Could you check a few things on this model? Use its own coordinates, in mm. Face numbers are marked on the shaded views. Round coordinates to 2 decimals unless told otherwise and drop trailing zeros. Loops run counter-clockwise (first coordinate to the right, second up) from the corner with the lowest first, then second, coordinate; pieces in that order, holes last. Notation, with made-up numbers: (81.5, -39) -> (129.5, -39) arc R34 ccw to (129.5, -7) -> close; hole circle Ø7 at (85, 79). An arc over 180 degrees is marked (long way). One line per item, written item: value.
```python
from build123d import *

# Parameters (mm, degrees)
SKETCH2_W = 20.317073171
SKETCH2_H = 3


with BuildPart() as part:
    # Sketch2 → Revolve1 (revolve)
    with BuildSketch(Plane(origin=(0, 0, 0), x_dir=(0, 0, -1), z_dir=(1, 0, 0)), mode=Mode.PRIVATE) as revolve1_sk:
        with Locations((5.158536586, -1.5)):
            Rectangle(SKETCH2_W, SKETCH2_H)
        Polygon((-5, 1.366666667), (-5, 0), (0, 0), align=None)
        Polygon((-5, 1.366666667), (0, 0), (7.317073171, 0), (-7.682926829, 4.1), (-7.682926829, 2.1), align=None)
        Polygon((19.317073171, -3), (15.317073171, -3), (15.317073171, 0), (19.317073171, -2.5), align=None)
    revolve(revolve1_sk.sketch.rotate(Axis((0, -3, 5), (0, 0, -1)), 180), axis=Axis((0, -3, 5), (0, 0, -1)))


solid = part.part
```
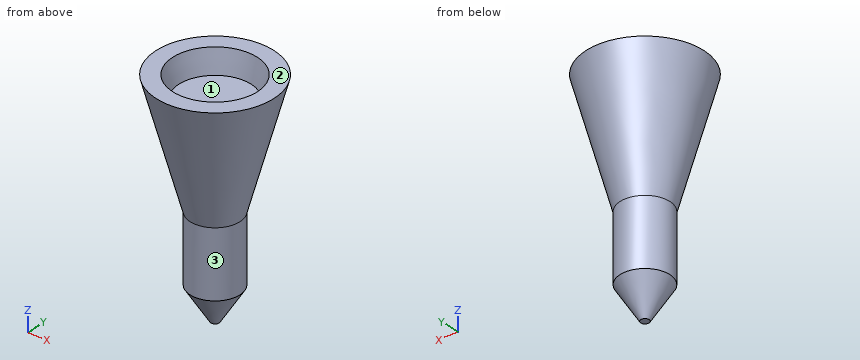
(1) Imagine slicing it at B-B on x = 0. Write out the boundary of the cut face in (y, z), then the cut area to 3 significant figures.
Results below:
outline: (-10.1, 7.68) -> (-6, -7.32) -> (-6, -15.32) -> (-3.5, -19.32) -> (-2.5, -19.32) -> (0, -15.32) -> (0, -7.32) -> (4.1, 7.68) -> (2.1, 7.68) -> (1.37, 5) -> (-7.37, 5) -> (-8.1, 7.68) -> close
area: 188 mm²
(2) Imagine slicing it at C-C on z = -12.75. Write out the boundary of the cut face in (x, y).
Results below:
outline: circle Ø6 at (0, -3)
(3) Please list where these lines run through material, in increasing order: L1, parallel to X at y = -4.25, z = 6; L2, parallel to Y at x = -5.25, z = 4; L3, parallel to X at y = 2.25, z = 4.5.
Results below:
L1: x = -6.52 to -4.47, 4.47 to 6.52
L2: y = -6.09 to 0.09
L3: x = -3.35 to 3.35
(4) For pin 1 Ø3 at (y, z) = (-7, -3) entering from +X; pin 2 Ø3 at (y, z) = (-2, -2) entering from +X; pin 3 Ø4 at (y, z) = (1.5, -1.5) entering from +X, each with a flat end and sliding along its axis, tell me the tip position at first contact or that it passes through.
Results below:
pin 1: stops at x = 3.46
pin 2: stops at x = 4.81
pin 3: stops at x = 4
(5) We'd pull the mould along Y, two halves only. Please class the marked faces 1, 2 and 3: +Y half, -Y half, draft (parallel to the pull), parting line (faces both ways), or undercut.
Results below:
face 1: undercut
face 2: draft
face 3: parting line
(6) Imagine slicing it at D-D on z = -4.5. Write out the boundary of the cut face in (x, y).
Results below:
outline: circle Ø7.54 at (0, -3)
(7) Imagine slicing it at A-A on y = -3. Write out the boundary of the cut face in (x, z), then the cut area to 3 significant figures.
Results below:
outline: (-7.1, 7.68) -> (-3, -7.32) -> (-3, -15.32) -> (-0.5, -19.32) -> (0.5, -19.32) -> (3, -15.32) -> (3, -7.32) -> (7.1, 7.68) -> (5.1, 7.68) -> (4.37, 5) -> (-4.37, 5) -> (-5.1, 7.68) -> close
area: 188 mm²
